Part model, mm, in its own coordinate system. A direction names the side the tool comes from. Round coordinates to 2 decimals unless told otherwise and drop trailing zeros. Write each loop counter-clockwise with the first axis right and the second up, starting at its lowest first coordinate (ties: lowest second). Pieces come first, ordered by that corner, then holes. Notation, with made-up numbers: M 0,41.25 L 56,41.25 A19 ccw 56,51.25 Z; hole C -4,-27.5 d3. An arc over 180 degrees is marked long. Answer as a JSON object with one key per item and string values. Group by question number.
1. Band-saw the part on B-B, the plane z = 16. Write the cut outline in (x, y).
2. Two-plate mould, pull along Y, no slides. Class faces 4 (the face through (0, 87, 10)), 5 (the face through (-10.46, 13.75, 4.93)), 6 (the face through (29.54, 13.75, 4.93)), 7 (the face through (-39, 4.5, 4.9)): +Y half, -Y half, draft (parallel to the pull), parting line (faces both ways), or undercut.
3. Band-saw the part on D-D, the plane y = 65. Write the cut outline in (x, z), plus the area to 3 significant figures.
4. Which spindle directions (+Z, -Z, +X, -X, +Y, -Y) get a long thin tool onto all of the face, cutting with end or side? Do faces 1 (the face through (-1, 22, 0)), 2 (the face through (0, 23.566, 20)), 3 (the face through (0, 70.751, 5)). Say none if no direction does.
5. Drop flat-ended pins along their axis: pin 1 (4 mm diameter, centred on y = 75, z = 43, fed in from +X); pin 2 (3 mm diameter, centred on x = 0.5, z = 16, fed in from -Y); pin 3 (12 mm diameter, centred on x = 20, y = 10.75, fed in from -Z); pin 4 (11 mm diameter, centred on x = -1.5, y = 88.5, fed in from -Z). Give the stop position or say it passes through.
6. Band-saw the part on C-C, the plane x = -14. Write the cut outline in (y, z).
7. Band-saw the part on A-A, the plane x = 14.5. Write the cut outline in (y, z).
8. Drill centre lines: line 1 (X direction, y = 72.5, z = 67); line 2 (Z direction, x = 10.5, y = 28); line 3 (Y direction, x = -20, z = 7). Where is each one in solid material? Low to high. Write a range as from..to.
from build123d import *

# Parameters (mm, degrees)
F0_R     = 10
F1_DEPTH = 10
F2_R     = 25
F3_R     = 25
F4_W     = 10
F4_H     = 79.0000073612
F5_DEPTH = 70
F6_R     = 50


with BuildPart() as f1:
    # F0 (on Top) → F1 (new body)
    with BuildSketch(Plane.XY):
        with BuildLine():
            Line((-5, 10.7507640496), (0, 10.7507640496))
            ThreePointArc((0, 10.7507640496), (-1.2917130661, 17.8218318615), (-5, 23.9795206049))
            Line((-5, 23.9795206049), (-5, 10.7507640496))
        make_face()
        with BuildLine():
            Line((5, 10.7507640496), (0, 10.7507640496))
            ThreePointArc((0, 10.7507640496), (20, -9.2492359504), (40, 10.7507640496))
            ThreePointArc((40, 10.7507640496), (27.0710678119, 29.4590509835), (5, 23.9795206049))
            Line((5, 23.9795206049), (5, 10.7507640496))
        make_face()
        with Locations((20, 10.7507640496)):
            Circle(F0_R, mode=Mode.SUBTRACT)
        with BuildLine():
            ThreePointArc((-5, 23.9795206049), (-1.2917130661, 17.8218318615), (0, 10.7507640496))
            ThreePointArc((0, 10.7507640496), (1.2917130661, 17.8218318615), (5, 23.9795206049))
            Line((5, 23.9795206049), (5, 70.7507640496))
            Line((5, 70.7507640496), (-5, 70.7507640496))
            Line((-5, 70.7507640496), (-5, 23.9795206049))
        make_face()
        with BuildLine():
            ThreePointArc((-5, 23.9795206049), (-38.7082869339, 3.6796962377), (0, 10.7507640496))
            Line((0, 10.7507640496), (-5, 10.7507640496))
            Line((-5, 10.7507640496), (-5, 23.9795206049))
        make_face()
        with Locations((-20, 10.7507640496)):
            Circle(F0_R, mode=Mode.SUBTRACT)
        with BuildLine():
            ThreePointArc((5, 23.9795206049), (1.2917130661, 17.8218318615), (0, 10.7507640496))
            Line((0, 10.7507640496), (5, 10.7507640496))
            Line((5, 10.7507640496), (5, 23.9795206049))
        make_face()
    extrude(amount=F1_DEPTH)

    # F2
    f2_edges = [f1.edges().sort_by_distance(p)[0] for p in [
        (0, 10.750764, 5),
    ]]
    fillet(f2_edges, radius=F2_R)

    # F3
    f3_edges = [f1.edges().sort_by_distance(p)[0] for p in [
        (-5, 23.979521, 5),
        (5, 23.979521, 5),
    ]]
    fillet(f3_edges, radius=F3_R)

    # F4 (on face) → F5 (join)
    with BuildSketch(Plane.XY.offset(10)):
        with Locations((0, 63.0660597235)):
            Rectangle(F4_W, F4_H)
    extrude(amount=F5_DEPTH)

    # F6
    f6_edges = [f1.edges().sort_by_distance(p)[0] for p in [
        (0, 23.566056, 80),
    ]]
    fillet(f6_edges, radius=F6_R)


solid = f1.part
Worked answers:
{
 "1": {"outline": "M -5,23.57 L 5,23.57 L 5,102.57 L -5,102.57 Z"},
 "2": {"face 4": "draft", "face 5": "undercut", "face 6": "undercut", "face 7": "parting line"},
 "3": {"outline": "M -5,0 L 5,0 L 5,79.26 L -5,79.26 Z", "area": "793 mm^2"},
 "4": {"face 1": "-Z, +X, -X, +Y, -Y", "face 2": "+Z, +X, -X, -Y", "face 3": "-Z, +X, -X, +Y"},
 "5": {"pin 1": "stops at x = 5", "pin 2": "stops at y = 23.57", "pin 3": "passes through", "pin 4": "stops at z = 10"},
 "6": {"outline": "M -8.33,0 L 2.75,0 L 2.75,10 L -8.33,10 Z; M 18.75,0 L 35.42,0 L 35.42,10 L 18.75,10 Z"},
 "7": {"outline": "M -8.48,0 L 2.4,0 L 2.4,10 L -8.48,10 Z; M 19.1,0 L 35.01,0 L 35.01,10 L 19.1,10 Z"},
 "8": {"line 1": "x = -5..5", "line 2": "z = 0..10", "line 3": "y = -9.25..0.75, 20.75..31.71"}
}
